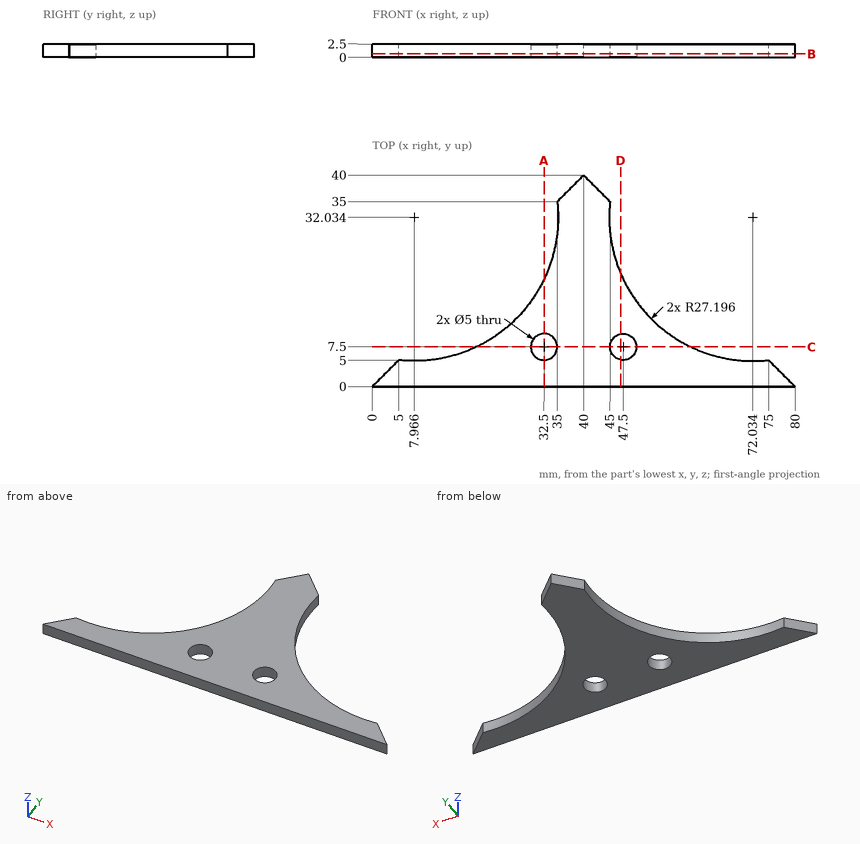
Design review of the part shown in the three views and the two pictorial views. Dimensions are in mm from the part's minimum x, y and z. Give positions to 0.01 mm unless a question says otherwise; leave off trailing zeros. Write each loop counter-clockwise with the first axis right and the second up, starting at its lowest first coordinate (ties: lowest second). Pieces come first, ordered by that corner, then holes. Notation, with made-up numbers: M 81,-4.5 L 99,-4.5 A16 ccw 99,23.5 Z; hole C 23.25,-29.75 d6. An arc over 180 degrees is marked long. One line per item, written item: value.
1) Take a section at D-D, the plane x = 47. Write out the cut boundary in (y, z), then the cut area to 3 significant figures.
Results are:
outline: M 0,0 L 5.05,0 L 5.05,2.5 L 0,2.5 Z; M 9.95,0 L 21.41,0 L 21.41,2.5 L 9.95,2.5 Z
area: 41.3 mm²
2) Take a section at B-B, the plane z = 0.65. Write out the cut boundary in (x, y), then the cut area to 3 significant figures.
Results are:
outline: M 0,0 L 80,0 L 75,5 A27.2 cw 45,35 L 40,40 L 35,35 A27.2 cw 5,5 Z; hole C 32.5,7.5 d5; hole C 47.5,7.5 d5
area: 959 mm²
3) For line 1 (X direction, y = 8.5, z = 0.75) (1 decimal); line 2 (Y direction, x = 5, z = 2.15); line 3 (Y direction, x = 47.5, z = 1.55), list the stretches that pass through material, from the lowest coordinate up. Write a range as from..to.
Results are:
line 1: x = 21.6..30.2, 34.8..45.2, 49.8..58.4
line 2: y = 0..5
line 3: y = 0..5, 10..20.3
4) For P1, Ø1.5, axis at x = 15, z = 1, coming from the +Y side; P2, Ø12, axis at x = 20.5, y = 22.5, coming from the +Z side, all flat-tipped, find the tip position at first contact; note any pin that passes through.
Results are:
P1: stops at y = 5.98
P2: passes through
5) Take a section at A-A, the plane x = 32.5. Write out the cut boundary in (y, z).
Results are:
outline: M 0,0 L 5,0 L 5,2.5 L 0,2.5 Z; M 10,0 L 20.3,0 L 20.3,2.5 L 10,2.5 Z
6) Take a section at C-C, the plane y = 7.5. Write out the cut boundary in (x, z).
Results are:
outline: M 19.7,0 L 30,0 L 30,2.5 L 19.7,2.5 Z; M 35,0 L 45,0 L 45,2.5 L 35,2.5 Z; M 50,0 L 60.3,0 L 60.3,2.5 L 50,2.5 Z
